The model under review builds one solid part; all positions refer to its coordinate system, in mm. A direction names the side the tool comes from. Give positions to 0.01 mm unless a question says otherwise; leave off trailing zeros. Order: outer loops, then holes, each group sorted by start corner. A loop starts at its lowest first (then second) coordinate and runs counter-clockwise, first axis right, second up.
```python
from build123d import *

# Parameters (mm, degrees)
F0_R           = 7.9248
F1_DEPTH       = 22.225
F3_D           = 3.175
F3_CSINK_D     = 6.35
F3_CSINK_ANGLE = 90
F4_R           = 6.35
F5_DEPTH       = 19.05
F6_SIZE        = 0.508
F7_SIZE        = 0.508


with BuildPart() as f1:
    # F0 (on Top) → F1 (new body)
    with BuildSketch(Plane.XY):
        Circle(F0_R)
    extrude(amount=-F1_DEPTH)

    # F3 (through all)
    with Locations(Plane.XY):
        with Locations((0, 0)):
            CounterSinkHole(F3_D / 2, F3_CSINK_D / 2, counter_sink_angle=F3_CSINK_ANGLE)

    # F4 (on face) → F5 (cut)
    with BuildSketch(Plane(origin=(0, 0, -22.225), x_dir=(1, 0, 0), z_dir=(0, 0, -1))):
        Circle(F4_R)
    extrude(amount=-F5_DEPTH, mode=Mode.SUBTRACT)

    # F6
    f6_edges = [f1.edges().sort_by_distance(p)[0] for p in [
        (-7.9248, 0, 0),
    ]]
    chamfer(f6_edges, length=F6_SIZE)

    # F7
    f7_edges = [f1.edges().sort_by_distance(p)[0] for p in [
        (-7.9248, 0, -22.225),
    ]]
    chamfer(f7_edges, length=F7_SIZE)


solid = f1.part
```
Item 1: For line 1 (Y direction, x = 0, z = -5.5); line 2 (X direction, y = -5, z = -6); line 3 (Y direction, x = -4.25, z = -15.25), list the stretches that pass through material, from the lowest coordinate up.
Values found:
line 1: y = -7.92 to -6.35, 6.35 to 7.92
line 2: x = -6.15 to -3.91, 3.91 to 6.15
line 3: y = -6.69 to -4.72, 4.72 to 6.69
Item 2: Clearance check with flat-ended pins moving along their axes: pin 1 Ø6 at (y, z) = (6, -18.5) entering from +X (3 decimals); pin 2 Ø1.5 at (x, z) = (3, -8) entering from +Y; pin 3 Ø6 at (x, z) = (-4, -9.5) entering from -Y. State where each tip first meets the part, or that it passes through.
Values found:
pin 1: stops at x = 7.335
pin 2: stops at y = 7.6
pin 3: stops at y = -7.86
Item 3: For faces 4 (the cylindrical face through (-1.38, 6.2, -12.83)), 5 (the flat face through (-3, 6, -22.225)), list the 3-axis set-ups (+Z, -Z, +X, -X, +Y, -Y) from which the entire face can be reached by the end or side of a thin tool; tool diameter is ignored.
Values found:
face 4: -Z
face 5: -Z, +X, -X, +Y, -Y
Item 4: Draft analysis for pull direction X (two halves, no side actions). For faces 1 (the cylindrical face through (-1.032, 7.857, -10.964)), 2 (the flat face through (1.3, 1.3, -3.175)), 3 (the flat face through (3, -2, 0)), state which applies: released by +X, released by -X, zero draft, split by the parting line, or undercut.
Values found:
face 1: split by the parting line
face 2: undercut
face 3: zero draft
Item 5: Take a section at D-D (z = -17.25). Give the boundary of the cut face in (x, y).
Values found:
outline: circle Ø15.85 at (0, 0); hole circle Ø12.7 at (0, 0)
Item 6: Take a section at C-C (z = -2.25). Give the boundary of the cut face in (x, y) (1 decimal).
Values found:
outline: circle Ø15.8 at (0, 0); hole circle Ø3.2 at (0, 0)
